from build123d import *

# Parameters (mm, degrees)
F0_R     = 3.5
F0_R_2   = 1.5
F1_DEPTH = 4
F2_R     = 2


with BuildPart() as f1:
    # F0 (on Top) → F1 (new body)
    with BuildSketch(Plane.XY):
        with BuildLine():
            Line((-12.5, -8.5), (-6, -16.3))
            Line((-6, -16.3), (0, -16.3))
            Line((0, -16.3), (6, -16.3))
            Line((6, -16.3), (12.5, -8.5))
            Line((12.5, -8.5), (13.5, 8.2))
            add(Edge.make_bspline(
                [(8.6, 16.7), (8.4917186517, 14.0737226405), (9.7758937627, 10.1948501542), (13.5, 8.2)],
                knots=[0, 0, 0, 0, 9.8112180691, 9.8112180691, 9.8112180691, 9.8112180691], degree=3))
            Line((8.6, 16.7), (11.5, 87.0371768306))
            Line((11.5, 87.0371768306), (7.3, 95.2371768306))
            ThreePointArc((7.3, 95.2371768306), (0, 99.7), (-7.3, 95.2371768306))
            Line((-7.3, 95.2371768306), (-11.5, 87.0371768306))
            Line((-11.5, 87.0371768306), (-8.6, 16.7))
            add(Edge.make_bspline(
                [(-8.6, 16.7), (-8.4917186517, 14.0737226405), (-9.7758937627, 10.1948501542), (-13.5, 8.2)],
                knots=[0, 0, 0, 0, 9.8112180691, 9.8112180691, 9.8112180691, 9.8112180691], degree=3))
            Line((-13.5, 8.2), (-12.5, -8.5))
        make_face()
        with BuildLine():
            Line((-7.2192388155, -5.3807611845), (-5.1686291501, -3.330151519))
            ThreePointArc((-5.1686291501, -3.330151519), (-3.330151519, -3.330151519), (-3.330151519, -5.1686291501))
            Line((-3.330151519, -5.1686291501), (-5.3807611845, -7.2192388155))
            ThreePointArc((-5.3807611845, -7.2192388155), (-7.2192388155, -7.2192388155), (-7.2192388155, -5.3807611845))
        make_face(mode=Mode.SUBTRACT)
        with BuildLine():
            ThreePointArc((-3.330151519, 5.1686291501), (-3.330151519, 3.330151519), (-5.1686291501, 3.330151519))
            Line((-5.1686291501, 3.330151519), (-7.2192388155, 5.3807611845))
            ThreePointArc((-7.2192388155, 5.3807611845), (-7.2192388155, 7.2192388155), (-5.3807611845, 7.2192388155))
            Line((-5.3807611845, 7.2192388155), (-3.330151519, 5.1686291501))
        make_face(mode=Mode.SUBTRACT)
        with BuildLine():
            Line((5.3807611845, -7.2192388155), (3.330151519, -5.1686291501))
            ThreePointArc((3.330151519, -5.1686291501), (3.330151519, -3.330151519), (5.1686291501, -3.330151519))
            Line((5.1686291501, -3.330151519), (7.2192388155, -5.3807611845))
            ThreePointArc((7.2192388155, -5.3807611845), (7.2192388155, -7.2192388155), (5.3807611845, -7.2192388155))
        make_face(mode=Mode.SUBTRACT)
        Circle(F0_R, mode=Mode.SUBTRACT)
        with BuildLine():
            Line((7.2192388155, 5.3807611845), (5.1686291501, 3.330151519))
            ThreePointArc((5.1686291501, 3.330151519), (3.330151519, 3.330151519), (3.330151519, 5.1686291501))
            Line((3.330151519, 5.1686291501), (5.3807611845, 7.2192388155))
            ThreePointArc((5.3807611845, 7.2192388155), (7.2192388155, 7.2192388155), (7.2192388155, 5.3807611845))
        make_face(mode=Mode.SUBTRACT)
        with Locations((-6, 80.0371768306)):
            Circle(F0_R_2, mode=Mode.SUBTRACT)
        with Locations((-6, 90.0371768306)):
            Circle(F0_R_2, mode=Mode.SUBTRACT)
        with Locations((6, 80.0371768306)):
            Circle(F0_R_2, mode=Mode.SUBTRACT)
        with Locations((6, 90.0371768306)):
            Circle(F0_R_2, mode=Mode.SUBTRACT)
    extrude(amount=F1_DEPTH)

    # F2
    f2_edges = [f1.edges().sort_by_distance(p)[0] for p in [
        (-11.5, 87.037177, 2),
        (11.5, 87.037177, 2),
        (13.5, 8.2, 2),
        (-13.5, 8.2, 2),
        (-12.5, -8.5, 2),
        (12.5, -8.5, 2),
        (6, -16.3, 2),
        (-6, -16.3, 2),
    ]]
    fillet(f2_edges, radius=F2_R)


solid = f1.part
For this review, take the finished solid that the model builds, in its own axes (mm). A direction names the side the tool comes from. Give positions to 0.01 mm unless a question says otherwise; leave off trailing zeros. Order: outer loops, then holes, each group sorted by start corner. A loop starts at its lowest first (then second) coordinate and runs counter-clockwise, first axis right, second up. Notation, with made-up numbers: M 70.25,77 L 107.25,77 A9 cw 107.25,86 Z; hole C -11.75,57 d7. An arc over 180 degrees is marked long. Answer in a Markdown table with one row per item. Add a question column.
(1) Consider section A-A on x = 0. State the section outline as (y, z) points, and give its area (3 significant figures).
(2) Mouldability with a two-part tool opening along X and no side actions: class faces 1 (the face through (0.1, 99.7, 2)), 2 (the face through (12.978, -0.523, 1.972)), 3 (the face through (6.18, -4.34, 1.97)) as +X half, -X half, draft (parallel to the pull), parting line (faces both ways), or undercut.
(3) For pin 1 (2.5 mm diameter, centred on x = 6, y = 90.04, fed in from +Z); pin 2 (1.5 mm diameter, centred on x = -0.5, y = 28, fed in from -Z); pin 3 (1.5 mm diameter, centred on y = 87, z = 1.5, fed in from +X); pin 4 (1 mm diameter, centred on y = 8, z = 1.5, fed in from -X), all flat-tipped, find the tip position at first contact; note any pin that passes through.
(4) For faces 4 (the face through (-4.37, 6.21, 1.97)), 5 (the face through (-12.99, -0.32, 1.97)), list the 3-axis set-ups (+Z, -Z, +X, -X, +Y, -Y) from which the entire face can be reached by the end or side of a thin tool; tool diameter is ignored.
(5) Wall thickness on probe 1 along Y at (x, z) = (6, 1.6); probe 2 along Y at (x, z) = (4, 1.95); probe 3 along X at (y, z) = (7, 0.2): over which ranges is each line inside the solid? List them lowest first. Write a range as [from, to].
(6) Consider section C-C on y = 28. State the section outline as (x, z) points, and give its area (3 significant figures).
(7) Consider section B-B on z = 1.65. Give the number of separate pieces and of enclosed holes in the cut face, and give its area (3 significant figures).
Evaluation:
| question | item | result |
|---|---|---|
| 1 | outline | M -16.3,0 L -3.5,0 L -3.5,4 L -16.3,4 Z; M 3.5,0 L 99.7,0 L 99.7,4 L 3.5,4 Z |
| 1 | area | 436 mm^2 |
| 2 | face 1 | parting line |
| 2 | face 2 | +X half |
| 2 | face 3 | undercut |
| 3 | pin 1 | passes through |
| 3 | pin 2 | stops at z = 0 |
| 3 | pin 3 | stops at x = 11.48 |
| 3 | pin 4 | stops at x = -13.4 |
| 4 | face 4 | +Z, -Z |
| 4 | face 5 | +Z, -Z, -X, -Y |
| 5 | probe 1 | y = [-16.07, -7.56], [-4.16, 4.16], [7.56, 78.54], [81.54, 88.54], [91.54, 97.09] |
| 5 | probe 2 | y = [-16.3, -5.84], [-2.97, 2.97], [5.84, 98.66] |
| 5 | probe 3 | x = [-13.43, -7.4], [-5.16, 5.16], [7.4, 13.43] |
| 6 | outline | M -9.07,0 L 9.07,0 L 9.07,4 L -9.07,4 Z |
| 6 | area | 72.5 mm^2 |
| 7 | separate pieces | 1 |
| 7 | enclosed holes | 9 |
| 7 | area | 2,240 mm^2 |
